Read the model definition and answer for the solid it produces. Units are mm, in the model's axes. Face numbers are marked on the shaded views. Coordinates: 2 decimals unless noted, no trailing zeros. Loops run counter-clockwise (first coordinate to the right, second up) from the corner with the lowest first, then second, coordinate; pieces in that order, holes last. Notation, with made-up numbers: (71.25, 36.5) -> (109.25, 36.5) arc R17 ccw to (109.25, 44.5) -> close; hole circle Ø1 at (-8.75, -28.75). An arc over 180 degrees is marked (long way). Answer in a Markdown table with one row per item.
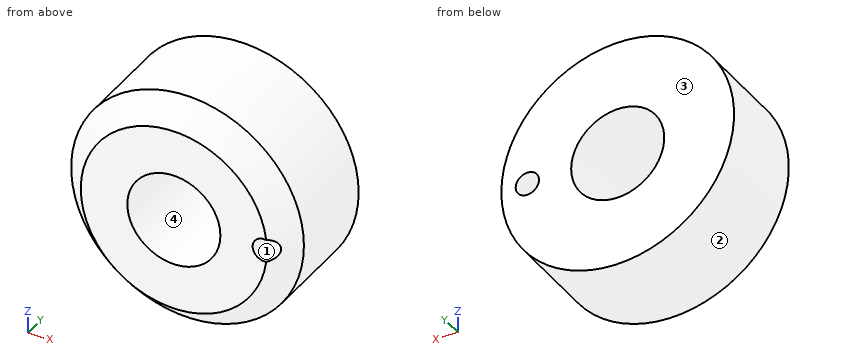
```python
from build123d import *

# Parameters (mm, degrees)
F0_R     = 25
F1_DEPTH = 25
F2_R     = 10
F3_DEPTH = 50
F4_SIZE  = 5
F5_R     = 2.5
F6_DEPTH = 25


with BuildPart() as f1:
    # F0 (on Front) → F1 (new body)
    with BuildSketch(Plane.XZ):
        Circle(F0_R)
    extrude(amount=F1_DEPTH)

    # F2 (on Front) → F3 (cut)
    with BuildSketch(Plane.XZ):
        Circle(F2_R)
    extrude(amount=F3_DEPTH, mode=Mode.SUBTRACT)

    # F4
    f4_edges = [f1.edges().sort_by_distance(p)[0] for p in [
        (-25, -25, 0),
    ]]
    chamfer(f4_edges, length=F4_SIZE)

    # F5 (on Front) → F6 (cut)
    with BuildSketch(Plane.XZ):
        with Locations((19.415321, 0)):
            Circle(F5_R)
    extrude(amount=F6_DEPTH, mode=Mode.SUBTRACT)


solid = f1.part
```
1. A cutting plane is placed at A-A on x = 0. Give the vertices of the cut face in (y, z), and give its area (3 significant figures).
A:
| item | result |
|---|---|
| outline | (-25, -20) -> (-20, -25) -> (0, -25) -> (0, -10) -> (-25, -10) -> close; (-25, 10) -> (0, 10) -> (0, 25) -> (-20, 25) -> (-25, 20) -> close |
| area | 725 mm2 |
2. The mould has two halves that part along X. Classify the marked faces 1, 2, 3 and 4: pulls with the +X half, pulls with the -X half, needs draft (parallel to the pull), parting line crosses it, or undercut.
A:
| item | result |
|---|---|
| face 1 | undercut |
| face 2 | parting line crosses it |
| face 3 | needs draft |
| face 4 | undercut |
3. A cutting plane is placed at C-C on z = 0. Give the vertices of the cut face in (x, y), and give its area (3 significant figures).
A:
| item | result |
|---|---|
| outline | (-25, -20) -> (-20, -25) -> (-10, -25) -> (-10, 0) -> (-25, 0) -> close; (10, -25) -> (16.92, -25) -> (16.92, 0) -> (10, 0) -> close; (21.92, -23.08) -> (25, -20) -> (25, 0) -> (21.92, 0) -> close |
| area | 602 mm2 |
4. Given pin 1 Ø8 at (x, y) = (5.5, -12) entering from +Z; pin 2 Ø2 at (y, z) = (-14.5, -10) entering from -X; pin 3 Ø1 at (x, y) = (18.5, -19.5) entering from -Z, each flat-ended and moving along its own axis, determine where each tip first touches the part or whether it passes through.
A:
| item | result |
|---|---|
| pin 1 | stops at z = 24.95 |
| pin 2 | stops at x = -23.32 |
| pin 3 | stops at z = -17.35 |
5. Find the intervals of material crossed by probe 1 along Z at (x, y) = (-8, -23.25); probe 2 along Z at (x, y) = (20.5, -15.5); probe 3 along Z at (x, y) = (15, -15), in increasing order.
A:
| item | result |
|---|---|
| probe 1 | z = -20.23 to -6, 6 to 20.23 |
| probe 2 | z = -14.31 to -2.25, 2.25 to 14.31 |
| probe 3 | z = -20 to 20 |
6. A cutting plane is placed at B-B on y = -5.75. Give the vertices of the cut face in (x, z).
A:
| item | result |
|---|---|
| outline | circle Ø50 at (0, 0); hole circle Ø20 at (0, 0); hole circle Ø5 at (19.42, 0) |
